```python
from build123d import *

# Parameters (mm, degrees)
BASE_FLANGE2_DEPTH = 101.6
SKETCH11_R         = 2.38125
CUT_EXTRUDE1_DEPTH = 114.990901501


# Sheet-metal steps are written as plain solids
with BuildPart() as part:
    # Sketch6 → Base-Flange2 (new body)
    with BuildSketch(Plane(origin=(0, 0, 0), x_dir=(1, 0, 0), z_dir=(0, 1, 0))):
        with BuildLine():
            Line((38.1, 0), (6.35, 0))
            ThreePointArc((6.35, 0), (1.859871939, 1.859871939), (0, 6.35))
            Line((0, 6.35), (0, 38.1))
            Line((0, 38.1), (3.175, 38.1))
            Line((3.175, 38.1), (3.175, 6.35))
            ThreePointArc((3.175, 6.35), (4.10493597, 4.10493597), (6.35, 3.175))
            Line((6.35, 3.175), (38.1, 3.175))
            Line((38.1, 3.175), (38.1, 0))
        make_face()
    extrude(amount=BASE_FLANGE2_DEPTH)

    # Sketch11 → Cut-Extrude1 (cut, through all)
    with BuildSketch(Plane(origin=(3.175, 0, 0), x_dir=(0, 0, -1), z_dir=(1, 0, 0))):
        with Locations((22.225, 88.9)):
            Circle(SKETCH11_R)
        with Locations((22.225, 12.7)):
            Circle(SKETCH11_R)
        with Locations((22.225, 50.8)):
            Circle(SKETCH11_R)
    extrude(amount=-CUT_EXTRUDE1_DEPTH, mode=Mode.SUBTRACT)


solid = part.part
```
Geometry check sheet. Reference: the model listing, model coordinates, mm. A direction names the side the tool comes from. Give positions to 0.01 mm unless a question says otherwise; leave off trailing zeros. Order: outer loops, then holes, each group sorted by start corner. A loop starts at its lowest first (then second) coordinate and runs counter-clockwise, first axis right, second up. Notation, with made-up numbers: (14, 26) - (62, 26) arc R18 ccw to (62, 31) - close; hole circle Ø9 at (53, 9.25). An arc over 180 degrees is marked (long way). Write item = value, one per line. Start each with the question number.
1) Section check C-C (z = -35). Enter the section's corners in (x, y) (3 decimals), then the cut area to 3 significant figures.
2) Gauge pin test, flat ends, axial feed: pin 1 Ø16 at (y, z) = (60, -27.5) entering from +X (3 decimals); pin 2 Ø4.5 at (y, z) = (50.8, -22.225) entering from +X; pin 3 Ø8 at (x, y) = (24, 31.5) entering from -Z (3 decimals). Record the tip position at first contact, or that the pin passes through.
3) Access from +Z, -Z, +X, -X, +Y, -Y to the whole of each face (thin tool, end or side, straight path). Record for faces 1 (the flat face through (22, 50, -3.175)), 2 (the flat face through (0, 50, -26)).
4) Draft check along Z on faces 3 (the flat face through (2, 50, -38.1)), 4 (the cylindrical face through (1.61, 91.26, -21.92)), 5 (the flat face through (38.1, 50, -2)), 6 (the cylindrical face through (1.61, 15.06, -21.92)). Enter one of: released by +Z, released by -Z, zero draft, split by the parting line, or undercut.
5) Section check B-B (x = 23.5). Enter the section's corners in (y, z) (3 decimals).
6) Scan lines: L1, parallel to Z at x = 6, y = 74.5; L2, parallel to X at y = 34, z = -7.5 (3 decimals); L3, parallel to X at y = 94, z = -2. Record each from-to range of solid material in increasing order.
7) Section check A-A (y = 50.8). Enter the section's corners in (x, z) (3 decimals), then the cut area to 3 significant figures.
Geometry check:
q1.outline = (0, 0) - (3.175, 0) - (3.175, 101.6) - (0, 101.6) - close
q1.area = 323 mm2
q2.pin_1 = 3.175
q2.pin_2 = through
q2.pin_3 = -3.175
q3.face_1 = -Z, +X, +Y, -Y
q3.face_2 = +Z, -Z, -X, +Y, -Y
q4.face_3 = released by -Z
q4.face_4 = undercut
q4.face_5 = zero draft
q4.face_6 = undercut
q5.outline = (0, -3.175) - (101.6, -3.175) - (101.6, 0) - (0, 0) - close
q6.L1 = -3.19 to -0.01
q6.L2 = 0 to 3.175
q6.L3 = 1.72 to 38.1
q7.outline = (0, -38.1) - (3.175, -38.1) - (3.175, -24.606) - (0, -24.606) - close; (0, -19.844) - (3.175, -19.844) - (3.175, -6.35) arc R3.175 cw to (6.35, -3.175) - (38.1, -3.175) - (38.1, 0) - (6.35, 0) arc R6.35 ccw to (0, -6.35) - close
q7.area = 210 mm2
